Geometry check sheet. Reference: the model listing, model coordinates, mm. A direction names the side the tool comes from. Round coordinates to 2 decimals unless told otherwise and drop trailing zeros. Write each loop counter-clockwise with the first axis right and the second up, starting at its lowest first coordinate (ties: lowest second). Pieces come first, ordered by that corner, then holes. Notation, with made-up numbers: (-26, 66) - (-14, 66) arc R22 cw to (-14, 88) - close; hole circle Ø8 at (29, 63.25). An arc over 180 degrees is marked (long way). Return JSON: item names as keys, results as strings.
```python
from build123d import *

# Parameters (mm, degrees)
SKETCH1_W           = 13.97
SKETCH1_H           = 213.36
BOSS_EXTRUDE1_DEPTH = 190.5
BOSS_EXTRUDE2_DEPTH = 50.8
SKETCH5_W           = 254
SKETCH5_H           = 254
BOSS_EXTRUDE3_DEPTH = 12.7
SKETCH6_W           = 228.6
SKETCH6_H           = 177.8
CUT_EXTRUDE1_DEPTH  = 12.7
SKETCH1_4_W         = 13.97
SKETCH1_4_H         = 213.36
BOSS_EXTRUDE5_DEPTH = 50.8
SKETCH8_W           = 12.7
SKETCH8_H           = 213.36
BOSS_EXTRUDE6_DEPTH = 50.8


with BuildPart() as part:
    # Sketch1 → Boss-Extrude1 (new body)
    with BuildSketch(Plane(origin=(0, 0, 0), x_dir=(1, 0, 0), z_dir=(0, 1, 0))):
        Polygon((0, 120.65), (0, 127), (-127, 127), (-127, -127), (0, -127), (0, -120.65), (-120.65, -120.65), (-120.65, -106.68), (-120.65, 106.68), (-120.65, 120.65), align=None)
        with Locations((-113.665, 0)):
            Rectangle(SKETCH1_W, SKETCH1_H)
        Polygon((127, 127), (0, 127), (0, 120.65), (120.65, 120.65), (120.65, 106.68), (120.65, -106.68), (120.65, -120.65), (0, -120.65), (0, -127), (127, -127), align=None)
        with Locations((113.665, 0)):
            Rectangle(SKETCH1_W, SKETCH1_H)
    extrude(amount=BOSS_EXTRUDE1_DEPTH)

    # Sketch4 → Boss-Extrude2 (add)
    with BuildSketch(Plane.XZ):
        Polygon((-127, 127), (-127, -127), (-120.65, -127), (-120.65, -120.65), (-120.65, -106.68), (-120.65, 106.68), (-120.65, 120.65), (120.65, 120.65), (120.65, 106.68), (120.65, -106.68), (120.65, -120.65), (120.65, -127), (127, -127), (127, 127), align=None)
    extrude(amount=BOSS_EXTRUDE2_DEPTH)

    # Sketch5 → Boss-Extrude3 (add)
    with BuildSketch(Plane.XZ.offset(50.8)):
        Rectangle(SKETCH5_W, SKETCH5_H)
    extrude(amount=BOSS_EXTRUDE3_DEPTH)

    # Sketch6 → Cut-Extrude1 (cut)
    with BuildSketch(Plane.XY.offset(127)):
        with Locations((0, 88.9)):
            Rectangle(SKETCH6_W, SKETCH6_H)
    extrude(amount=-CUT_EXTRUDE1_DEPTH, mode=Mode.SUBTRACT)

    # Sketch1_4 → Boss-Extrude5 (add)
    with BuildSketch(Plane(origin=(0, 0, 0), x_dir=(1, 0, 0), z_dir=(0, 1, 0))):
        with Locations((113.665, 0)):
            Rectangle(SKETCH1_4_W, SKETCH1_4_H)
        with Locations((-113.665, 0)):
            Rectangle(SKETCH1_4_W, SKETCH1_4_H)
    extrude(amount=-BOSS_EXTRUDE5_DEPTH)

    # Sketch8 → Boss-Extrude6 (add)
    with BuildSketch(Plane(origin=(0, -50.8, 0), x_dir=(1, 0, 0), z_dir=(0, 1, 0))):
        with Locations((-100.33, 0)):
            Rectangle(SKETCH8_W, SKETCH8_H)
        with Locations((100.33, 0)):
            Rectangle(SKETCH8_W, SKETCH8_H)
    extrude(amount=BOSS_EXTRUDE6_DEPTH)


solid = part.part
```
(1) Gauge pin test, flat ends, axial feed: pin 1 (2 mm diameter, centred on x = -79.5, y = 33.5, fed in from +Z); pin 2 (3 mm diameter, centred on x = 8.5, z = 95, fed in from +Y); pin 3 (21.5 mm diameter, centred on x = -103.5, y = 73, fed in from +Z). Record the tip position at first contact, or that the pin passes through.
Response values:
{"pin 1": "stops at z = -120.65", "pin 2": "stops at y = -50.8", "pin 3": "stops at z = 106.68"}
(2) Section check A-A, the plane x = 56. Enter the section's corners in (y, z), plus the area to 3 significant figures.
Response values:
{"outline": "(-63.5, -127) - (-50.8, -127) - (-50.8, 120.65) - (0, 120.65) - (0, 127) - (-63.5, 127) - close; (0, -127) - (190.5, -127) - (190.5, -120.65) - (0, -120.65) - close; (177.8, 120.65) - (190.5, 120.65) - (190.5, 127) - (177.8, 127) - close", "area": "4,840 mm^2"}
(3) Material ranges on line 1 along X through (y, z) = (13, -3.5); line 2 along X through (y, z) = (-41, -110.5); line 3 along Z through (x, y) = (-115, -45), recorded low to high. Write a range as [from, to].
Response values:
{"line 1": "x = [-127, -106.68], [106.68, 127]", "line 2": "x = [-127, -120.65], [120.65, 127]", "line 3": "z = [-106.68, 106.68], [120.65, 127]"}
(4) Section check B-B, the plane z = -55.5. Enter the section's corners in (x, y).
Response values:
{"outline": "(-127, -63.5) - (127, -63.5) - (127, 190.5) - (106.68, 190.5) - (106.68, 0) - (93.98, 0) - (93.98, -50.8) - (-93.98, -50.8) - (-93.98, 0) - (-106.68, 0) - (-106.68, 190.5) - (-127, 190.5) - close"}
(5) Release check for a two-part mould opening along Z. For faces 1 (the face through (-2, 94, -127)), 2 (the face through (100, 0, -1)), 3 (the face through (-120.65, 72, -115)) record: pulls with the +Z half, pulls with the -Z half, needs draft (parallel to the pull), parting line crosses it, or undercut.
Response values:
{"face 1": "pulls with the -Z half", "face 2": "needs draft", "face 3": "undercut"}
(6) Section check C-C, the plane y = 23. Enter the section's corners in (x, z).
Response values:
{"outline": "(-127, -127) - (127, -127) - (127, 127) - (114.3, 127) - (114.3, 120.65) - (120.65, 120.65) - (120.65, 106.68) - (106.68, 106.68) - (106.68, -106.68) - (120.65, -106.68) - (120.65, -120.65) - (-120.65, -120.65) - (-120.65, -106.68) - (-106.68, -106.68) - (-106.68, 106.68) - (-120.65, 106.68) - (-120.65, 120.65) - (-114.3, 120.65) - (-114.3, 127) - (-127, 127) - close"}
(7) Access from +Z, -Z, +X, -X, +Y, -Y to the whole of each face (thin tool, end or side, straight path). Record for faces 4 (the face through (-2, -63.5, 2)), 5 (the face through (-93.98, -26, 1)), 6 (the face through (110, 45, 106.68)).
Response values:
{"face 4": "+Z, -Z, +X, -X, -Y", "face 5": "-Z, +Y", "face 6": "+Y"}
